from build123d import *

# Parameters (mm, degrees)
F0_R     = 12.7
F0_R_2   = 6.35
F1_DEPTH = 25.4
F2_R     = 21.59
F2_R_2   = 12.7
F3_DEPTH = 12.7


with BuildPart() as f1:
    # F0 (on Top) → F1 (new body)
    with BuildSketch(Plane.XY):
        with Locations((0, 39.825506)):
            Circle(F0_R)
        with Locations((0, 39.825506)):
            Circle(F0_R_2, mode=Mode.SUBTRACT)
    extrude(amount=F1_DEPTH)

    # F2 (on face) → F3 (join)
    with BuildSketch(Plane.XY.offset(25.4)):
        with Locations((0, 39.825506)):
            Circle(F2_R)
        with Locations((0, 39.825506)):
            Circle(F2_R_2, mode=Mode.SUBTRACT)
    extrude(amount=-F3_DEPTH)


with BuildPart() as f1_1:
    # F4: moved
    add(f1.part.moved(Location((0, -40.64, 0))))


solid = f1_1.part
Read the model definition and answer for the solid it produces. Units are mm, in the model's axes. A direction names the side the tool comes from. Coordinates: 2 decimals unless noted, no trailing zeros. Loops run counter-clockwise (first coordinate to the right, second up) from the corner with the lowest first, then second, coordinate; pieces in that order, holes last. Notation, with made-up numbers: (15, 22) -> (47, 22) arc R20 ccw to (47, 45) -> close; hole circle Ø3 at (-5.75, -27). An arc over 180 degrees is marked (long way). Answer in a Markdown table with one row per item.
Item 1: Each of these flat-tipped pins is pushed along its axis until it touches: P1, Ø8, axis at y = -15.5, z = 22, coming from the -X side; P2, Ø8, axis at x = 4, z = 4.5, coming from the -Y side; P3, Ø12, axis at x = -14.5, y = -13.5, coming from the -Z side. Where does it stop, or does it pass through?
Returned:
| item | result |
|---|---|
| P1 | stops at x = -18.76 |
| P2 | stops at y = -13.51 |
| P3 | stops at z = 12.7 |
Item 2: A cutting plane is placed at B-B on y = 3.5. Determine the outline of the cut face in (x, z), plus the area to 3 significant figures.
Returned:
| item | result |
|---|---|
| outline | (-21.15, 12.7) -> (-11.94, 12.7) -> (-11.94, 0) -> (-4.66, 0) -> (-4.66, 25.4) -> (-21.15, 25.4) -> close; (4.66, 0) -> (11.94, 0) -> (11.94, 12.7) -> (21.15, 12.7) -> (21.15, 25.4) -> (4.66, 25.4) -> close |
| area | 604 mm^2 |
Item 3: Straight lines are drawn through the part: line 1 along Y through (x, z) = (0, 18); line 2 along Y through (x, z) = (0, 11.5); line 3 along Z through (x, y) = (-17.5, -4.5). For each, find the intervals that lie inside material, in ascending order. Write a range as [from, to].
Returned:
| item | result |
|---|---|
| line 1 | y = [-22.4, -7.16], [5.54, 20.78] |
| line 2 | y = [-13.51, -7.16], [5.54, 11.89] |
| line 3 | z = [12.7, 25.4] |
Item 4: For a pull along Y with two mould halves and no side action, classify faces 3 (the cylindrical face through (-0.83, 5.48, 12.52)), 4 (the cylindrical face through (-17.133, -13.952, 19.139)), 5 (the flat face through (3, 5, 0)) as released by +Y, released by -Y, zero draft, split by the parting line, or undercut.
Returned:
| item | result |
|---|---|
| face 3 | undercut |
| face 4 | split by the parting line |
| face 5 | zero draft |
Item 5: For faces 1 (the flat face through (-5, -5, 25.4)), 2 (the cylindrical face through (-2.8, -13.2, 6.3)), determine the directions among +Z, -Z, +X, -X, +Y, -Y from which every point of the face is accessible in a straight line to the end or side of a thin tool.
Returned:
| item | result |
|---|---|
| face 1 | +Z, +X, -X, +Y, -Y |
| face 2 | -Z |
Item 6: A cutting plane is placed at A-A on x = 0. Determine the outline of the cut face in (y, z), plus the area to 3 significant figures.
Returned:
| item | result |
|---|---|
| outline | (-22.4, 12.7) -> (-13.51, 12.7) -> (-13.51, 0) -> (-7.16, 0) -> (-7.16, 25.4) -> (-22.4, 25.4) -> close; (5.54, 0) -> (11.89, 0) -> (11.89, 12.7) -> (20.78, 12.7) -> (20.78, 25.4) -> (5.54, 25.4) -> close |
| area | 548 mm^2 |
Item 7: A cutting plane is placed at D-D on z = 20.5. Determine the outline of the cut face in (x, y).
Returned:
| item | result |
|---|---|
| outline | circle Ø43.18 at (0, -0.81); hole circle Ø12.7 at (0, -0.81) |
Item 8: A cutting plane is placed at C-C on x = -10.5. Determine the outline of the cut face in (y, z), plus the area to 3 significant figures.
Returned:
| item | result |
|---|---|
| outline | (-19.68, 12.7) -> (-7.96, 12.7) -> (-7.96, 0) -> (6.33, 0) -> (6.33, 12.7) -> (18.05, 12.7) -> (18.05, 25.4) -> (-19.68, 25.4) -> close |
| area | 661 mm^2 |
